Here's the drawing with two shaded views (mm, measured from the low corner). I have some questions. Give positions to 0.01 mm unless a question says otherwise; leave off trailing zeros. Loops run counter-clockwise (first coordinate to the right, second up) from the corner with the lowest first, then second, coordinate; pieces in that order, holes last. Notation, with made-up numbers: M 72,37 L 97,37 A26 ccw 97,64 Z; hole C 29,26 d11. An arc over 180 degrees is marked long. Write item = value, one per line. Start each with the question number.
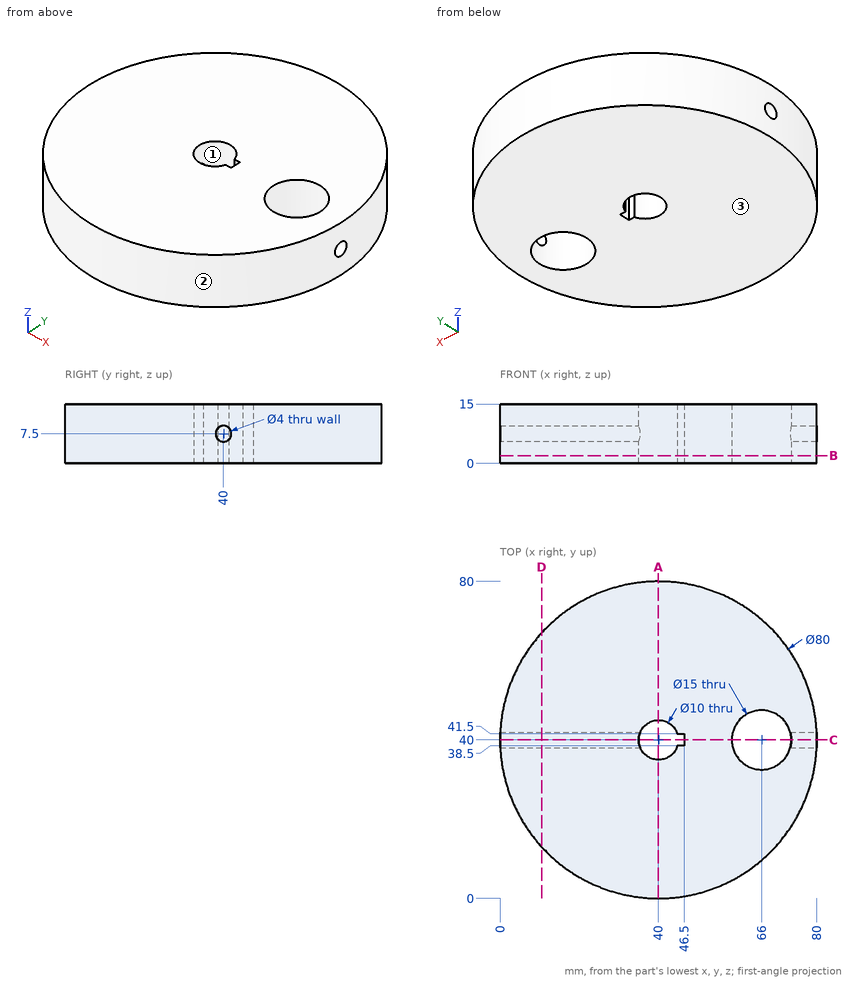
Q1. If we section it at D-D, the plane x = 10.5: List the corners of the cut face in (y, z) for me, then the cut area to 3 significant figures.
Q2. If we section it at C-C, the plane y = 40: List the corners of the cut face in (x, z) for me.
Q3. If we section it at A-A, the plane x = 40: List the corners of the cut face in (y, z) for me, then the cut area to 3 significant figures.
Q4. If I drill on line 1 along Y through (x, z) = (40, 5); line 2 along X through (y, z) = (41, 9.5); line 3 along X through (y, z) = (34, 7.25), over which ranges is the centre line in solid material (lowest first)?
Q5. If we section it at B-B, the plane z = 2: List the corners of the cut face in (x, y) for me, then the cut area to 3 significant figures.
Q6. We'd pull the mould along X, two halves only. Please class the marked faces 1, 2 and 3: pulls with the +X half, pulls with the -X half, needs draft (parallel to the pull), parting line crosses it, or undercut.
Q7. Will these pins go through, and if not, where does the flat tip stop? pin 1 (4 mm diameter, centred on y = 66.5, z = 3, fed in from +X); pin 2 (2 mm diameter, centred on x = 15, z = 4, fed in from -Y); pin 3 (0.5 mm diameter, centred on x = 46, z = 4.5, fed in from -Y); pin 4 (4.5 mm diameter, centred on y = 40, z = 7.5, fed in from -X).
Resolved:
q1.outline = M 12.99,0 L 67.01,0 L 67.01,15 L 12.99,15 Z; hole C 40,7.5 d4
q1.area = 798 mm²
q2.outline = M 0,0 L 35,0 L 35,5.5 L 0,5.5 Z; M 0,9.5 L 35,9.5 L 35,15 L 0,15 Z; M 46.5,0 L 58.5,0 L 58.5,15 L 46.5,15 Z; M 73.5,0 L 80,0 L 80,5.5 L 73.5,5.5 Z; M 73.5,9.5 L 80,9.5 L 80,15 L 73.5,15 Z
q3.outline = M 0,0 L 35,0 L 35,15 L 0,15 Z; M 45,0 L 80,0 L 80,15 L 45,15 Z
q3.area = 1,050 mm²
q4.line_1 = 0 to 35, 45 to 80
q4.line_2 = 0.01 to 35.1, 46.5 to 58.57, 73.43 to 79.99
q4.line_3 = 0.45 to 61.5, 70.5 to 79.55
q5.outline = C 40,40 d80; hole M 44.77,38.5 L 46.5,38.5 L 46.5,41.5 L 44.77,41.5 A5 ccw long Z; hole C 66,40 d15
q5.area = 4,770 mm²
q6.face_1 = undercut
q6.face_2 = parting line crosses it
q6.face_3 = needs draft
q7.pin_1 = 71.62
q7.pin_2 = 8
q7.pin_3 = 0.42
q7.pin_4 = 0
